Part print with two shaded views. Sizes in mm from the minimum x, y, z corner. A direction names the side the tool comes from. Give positions to 0.01 mm unless a question says otherwise; leave off trailing zeros. Write each loop counter-clockwise with the first axis right and the second up, starting at its lowest first coordinate (ties: lowest second). Pieces come first, ordered by that corner, then holes.
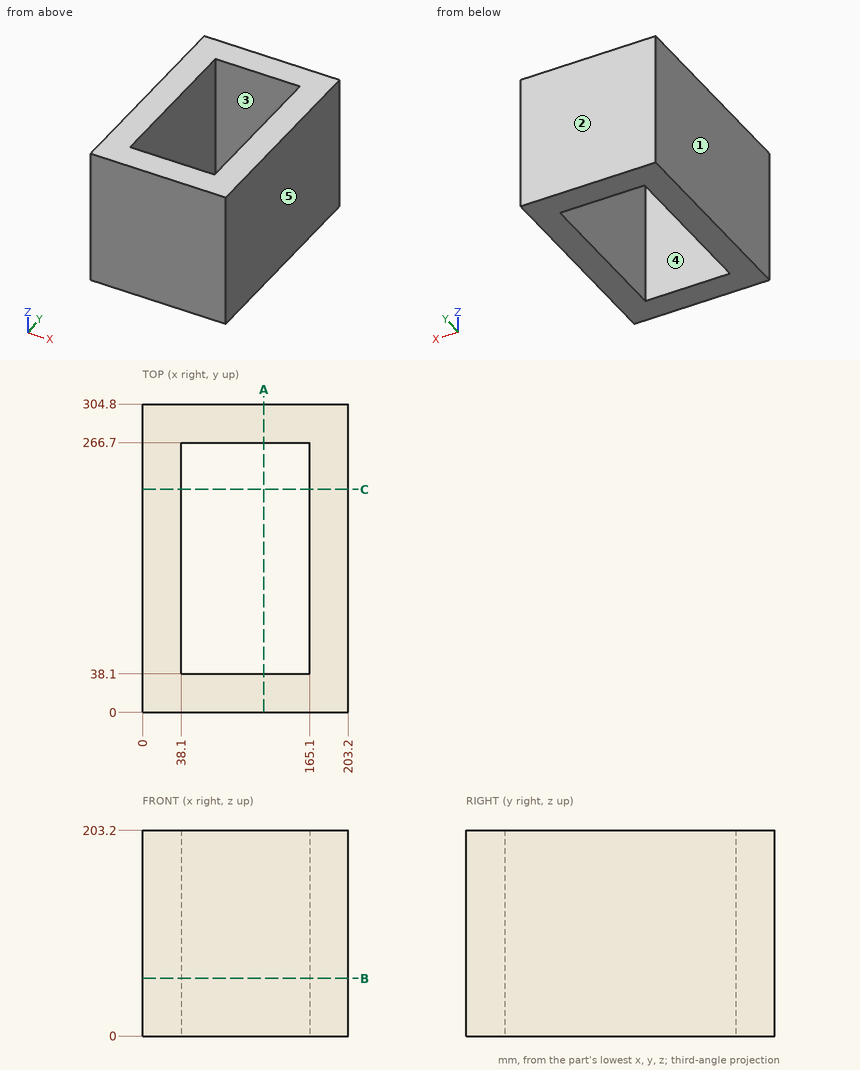
1) 3-axis set-ups, long thin cutter, end or side, ignore diameter. For the marked faces 4 and 5: which of +Z, -Z, +X, -X, +Y, -Y reach the whole face in a straight line?
Check result:
face 4: +Z, -Z
face 5: +Z, -Z, +X, +Y, -Y
2) Saw through at B-B (z = 57). Write the cut outline in (x, y), and give its area (3 significant figures).
Check result:
outline: (0, 0) - (203.2, 0) - (203.2, 304.8) - (0, 304.8) - close; hole (38.1, 38.1) - (165.1, 38.1) - (165.1, 266.7) - (38.1, 266.7) - close
area: 32,900 mm2
3) Flat gauge pin, fed straight in: P1, Ø5, axis at x = 81.5, y = 262, coming from the +Z side. Where does the tip first touch, or does it go through?
Check result:
P1: passes through
4) Mould opens along X. For the marked faces 1, 2 and 3 say: +X half, -X half, draft (parallel to the pull), parting line (faces both ways), or undercut.
Check result:
face 1: -X half
face 2: draft
face 3: undercut
5) Saw through at C-C (y = 220.5). Write the cut outline in (x, z).
Check result:
outline: (0, 0) - (38.1, 0) - (38.1, 203.2) - (0, 203.2) - close; (165.1, 0) - (203.2, 0) - (203.2, 203.2) - (165.1, 203.2) - close
6) Saw through at A-A (x = 120). Write the cut outline in (y, z).
Check result:
outline: (0, 0) - (38.1, 0) - (38.1, 203.2) - (0, 203.2) - close; (266.7, 0) - (304.8, 0) - (304.8, 203.2) - (266.7, 203.2) - close
7) Drill centre lines: L1, parallel to X at y = 85.5, z = 85.5; L2, parallel to Y at x = 53.5, z = 143. Where is each one in solid material? Low to high.
Check result:
L1: x = 0 to 38.1, 165.1 to 203.2
L2: y = 0 to 38.1, 266.7 to 304.8
